Design review of the part built by this model. Coordinates are the model's own, in mm. A direction names the side the tool comes from. Round coordinates to 2 decimals unless told otherwise and drop trailing zeros. Order: outer loops, then holes, each group sorted by start corner. A loop starts at its lowest first (then second) coordinate and runs counter-clockwise, first axis right, second up. Notation, with made-up numbers: (61, 16.5) - (89, 16.5) arc R10 cw to (89, 32.5) - close; hole circle Ø1 at (48, 88.5). An arc over 180 degrees is marked (long way). Use CSV: the item, a comma, the result in double quotes.
from build123d import *

# Parameters (mm, degrees)
BOSS_EXTRUDE1_DEPTH = 120
SKETCH3_W           = 44
SKETCH3_H           = 14
CUT_EXTRUDE2_DEPTH  = 30
SKETCH6_R           = 2.5
CUT_EXTRUDE3_DEPTH  = 30


with BuildPart() as part:
    # Sketch1 → Boss-Extrude1 (new body)
    with BuildSketch(Plane(origin=(0, 0, 0), x_dir=(1, 0, 0), z_dir=(0, 1, 0))):
        with BuildLine():
            Line((2, 0), (48, 0))
            ThreePointArc((48, 0), (49.414213562, 0.585786438), (50, 2))
            Line((50, 2), (50, 18))
            ThreePointArc((50, 18), (49.414213562, 19.414213562), (48, 20))
            Line((48, 20), (2, 20))
            ThreePointArc((2, 20), (0.585786438, 19.414213562), (0, 18))
            Line((0, 18), (0, 2))
            ThreePointArc((0, 2), (0.585786438, 0.585786438), (2, 0))
        make_face()
    extrude(amount=BOSS_EXTRUDE1_DEPTH)

    # Sketch3 → Cut-Extrude2 (cut)
    with BuildSketch(Plane.XZ):
        with Locations((25, -10)):
            Rectangle(SKETCH3_W, SKETCH3_H)
    extrude(amount=-CUT_EXTRUDE2_DEPTH, mode=Mode.SUBTRACT)

    # Sketch6 → Cut-Extrude3 (cut)
    with BuildSketch(Plane.XY):
        with Locations((25, 105)):
            Circle(SKETCH6_R)
        with Locations((25, 15)):
            Circle(SKETCH6_R)
    extrude(amount=-CUT_EXTRUDE3_DEPTH, mode=Mode.SUBTRACT)


solid = part.part
1) We need section C-C (y = 28). Give the boundary of the cut face in (x, z).
Data:
outline,"(0, -18) arc R2 ccw to (2, -20) - (48, -20) arc R2 ccw to (50, -18) - (50, -2) arc R2 ccw to (48, 0) - (2, 0) arc R2 ccw to (0, -2) - close; hole (3, -17) - (47, -17) - (47, -3) - (3, -3) - close"
2) For faces 4 (the face through (3, 15, -10)), 5 (the face through (0.57, 59.16, -0.6)), list the 3-axis set-ups (+Z, -Z, +X, -X, +Y, -Y) from which the entire face can be reached by the end or side of a thin tool; tool diameter is ignored.
Data:
face 4,"-Y"
face 5,"+Z, -X, +Y, -Y"
3) We need section D-D (x = 25). Give the boundary of the cut face in (y, z).
Data:
outline,"(0, -20) - (12.5, -20) - (12.5, -17) - (0, -17) - close; (0, -3) - (12.5, -3) - (12.5, 0) - (0, 0) - close; (17.5, -20) - (102.5, -20) - (102.5, 0) - (17.5, 0) - (17.5, -3) - (30, -3) - (30, -17) - (17.5, -17) - close; (107.5, -20) - (120, -20) - (120, 0) - (107.5, 0) - close"
4) The part is to be moulded in two halves that separate along Z. For faces 1 (the face through (25, 11, -17)), 2 (the face through (25, 59, -20)), 3 (the face through (0, 59, -10)), say which applies: +Z half, -Z half, draft (parallel to the pull), parting line (faces both ways), or undercut.
Data:
face 1,"undercut"
face 2,"-Z half"
face 3,"draft"
5) To check wall thickness, follow L1, parallel to Y at x = 25, z = -6.25; L2, parallel to Z at x = 30.5, y = 28; L3, parallel to Y at x = 25, z = -18.7. State the ranges of each line that lie inside material, in increasing order. Write a range as from..to.
Data:
L1,"y = 30..102.5, 107.5..120"
L2,"z = -20..-17, -3..0"
L3,"y = 0..12.5, 17.5..102.5, 107.5..120"
6) Insertion check: pin 1 Ø3 at (x, y) = (25, 15) entering from -Z; pin 2 Ø10 at (x, z) = (19.5, -11) entering from -Y. Each pin has a flat end and moves straight along its axis. Give the tip position at first contact, or say it passes through.
Data:
pin 1,"passes through"
pin 2,"stops at y = 30"
7) We need section B-B (z = -10.75). Give the boundary of the cut face in (x, y).
Data:
outline,"(0, 0) - (3, 0) - (3, 30) - (47, 30) - (47, 0) - (50, 0) - (50, 120) - (0, 120) - close; hole circle Ø5 at (25, 105)"
8) We need section A-A (y = 105). Give the boundary of the cut face in (x, z), then the cut area to 3 significant figures.
Data:
outline,"(0, -18) arc R2 ccw to (2, -20) - (22.5, -20) - (22.5, 0) - (2, 0) arc R2 ccw to (0, -2) - close; (27.5, -20) - (48, -20) arc R2 ccw to (50, -18) - (50, -2) arc R2 ccw to (48, 0) - (27.5, 0) - close"
area,"897 mm2"
